from build123d import *

# Parameters (mm, degrees)
F0_W     = 58
F0_H     = 85
F1_DEPTH = 35
F2_W     = 57.238
F2_H     = 19.05
F3_DEPTH = 28.448
F4_W     = 31.75
F4_H     = 9.525
F5_DEPTH = 9.525
F7_D     = 1.27
F7_DEPTH = 5.08
F7_TIP   = 0.3815464931


with BuildPart() as f1:
    # F0 (on Top) → F1 (new body)
    with BuildSketch(Plane.XY):
        Rectangle(F0_W, F0_H)
    extrude(amount=F1_DEPTH)

    # F2 (on face) → F3 (cut)
    with BuildSketch(Plane.XY.offset(35)):
        with Locations((-0.381, -32.975)):
            Rectangle(F2_W, F2_H)
    extrude(amount=-F3_DEPTH, mode=Mode.SUBTRACT)

    # F4 (on face) → F5 (join)
    with BuildSketch(Plane.XY.offset(6.552)):
        with Locations((-0.381, -36.4675)):
            Rectangle(F4_W, F4_H)
    extrude(amount=F5_DEPTH)

    # F7
    with Locations(Plane.XZ.offset(41.23)):
        with Locations((-10.9643333333, 11.3145), (-5.6726666667, 11.3145), (-0.381, 11.3145), (4.9106666667, 11.3145), (10.2023333333, 11.3145)):
            Hole(F7_D / 2, depth=F7_DEPTH)
            with Locations((0, 0, -(F7_DEPTH + F7_TIP / 2))):  # 118° drill point
                Cone(0, F7_D / 2, F7_TIP, mode=Mode.SUBTRACT)


solid = f1.part
Here's how the part is built. I have some questions about the finished solid (model axes, mm). A direction names the side the tool comes from. Coordinates: 2 decimals unless noted, no trailing zeros. Order: outer loops, then holes, each group sorted by start corner. A loop starts at its lowest first (then second) coordinate and runs counter-clockwise, first axis right, second up. Notation, with made-up numbers: M 8.25,15.5 L 25.25,15.5 A22 cw 25.25,43.5 Z; hole C -9.75,74 d5. An arc over 180 degrees is marked long. Answer as CSV lines item,"result". Start each with the question number.
1. I want a section at C-C, the plane y = -33. Write out the boundary of the cut face in (x, z), and give its area (3 significant figures).
2. I want a section at B-B, the plane x = 6.5. Write out the boundary of the cut face in (y, z) (3 decimals).
3. I need wall thicknesses on line 1 (Y direction, x = 5.5, z = 16) (3 decimals); line 2 (Z direction, x = 5, y = -38.5); line 3 (X direction, y = -37.5, z = 8.5). Which ranges of each line are inside material? Lowest first, please. Write a range as [from, to].
4. On a 3-axis mill with a long thin cutter (end or side, diameter ignored), from which of +Z, -Z, +X, -X, +Y, -Y can I reach the whole of each face in a straight line? I mean faces 4 (the flat face through (0, -42.5, 3)), 5 (the flat face through (-1, -31.705, 11)), 6 (the flat face through (15.494, -37, 11)), 7 (the flat face through (-16.256, -37, 11)). Say none if no direction works.
5. For pin 1 (14 mm diameter, centred on x = 2, z = 18, fed in from -Y); pin 2 (4 mm diameter, centred on x = 18.5, y = -32.5, fed in from +Z); pin 3 (0.8 mm diameter, centred on x = -0.38, z = 11.31, fed in from -Y), each with a flat end and sliding along its axis, tell me the tip position at first contact or that it passes through.
6. I want a section at D-D, the plane z = 22. Write out the boundary of the cut face in (x, y).
7. We'd pull the mould along Y, two halves only. Please class faces 1 (the flat face through (-1, -31, 6.552)), 2 (the flat face through (0, 42.5, 17)), 3 (the flat face through (0, 10, 35)): released by +Y, released by -Y, zero draft, split by the parting line, or undercut.
8. I want a section at A-A, the plane z = 15. Write out the boundary of the cut face in (x, y) (3 decimals), and give its area (3 significant figures).
Recorded:
1,outline,"M -29,0 L 29,0 L 29,35 L 28.24,35 L 28.24,6.55 L 15.49,6.55 L 15.49,16.08 L -16.26,16.08 L -16.26,6.55 L -29,6.55 Z"
1,area,"704 mm2"
2,outline,"M -42.5,0 L 42.5,0 L 42.5,35 L -23.45,35 L -23.45,6.552 L -31.705,6.552 L -31.705,16.077 L -41.23,16.077 L -41.23,6.552 L -42.5,6.552 Z"
3,line 1,"y = [-41.23, -31.705], [-23.45, 42.5]"
3,line 2,"z = [0, 10.69], [11.94, 16.08]"
3,line 3,"x = [-16.26, 15.49], [28.24, 29]"
4,face 4,"+Z, -Z, +X, -X, -Y"
4,face 5,"+Z, -X"
4,face 6,"+Z, -Y"
4,face 7,"+Z, -X, -Y"
5,pin 1,"stops at y = -41.23"
5,pin 2,"stops at z = 6.55"
5,pin 3,"stops at y = -36.01"
6,outline,"M -29,-23.45 L 28.24,-23.45 L 28.24,-42.5 L 29,-42.5 L 29,42.5 L -29,42.5 Z"
7,face 1,"undercut"
7,face 2,"released by +Y"
7,face 3,"zero draft"
8,outline,"M -29,-23.45 L 28.238,-23.45 L 28.238,-42.5 L 29,-42.5 L 29,42.5 L -29,42.5 Z; M -16.256,-41.23 L 15.494,-41.23 L 15.494,-31.705 L -16.256,-31.705 Z"
8,area,"4,140 mm2"
